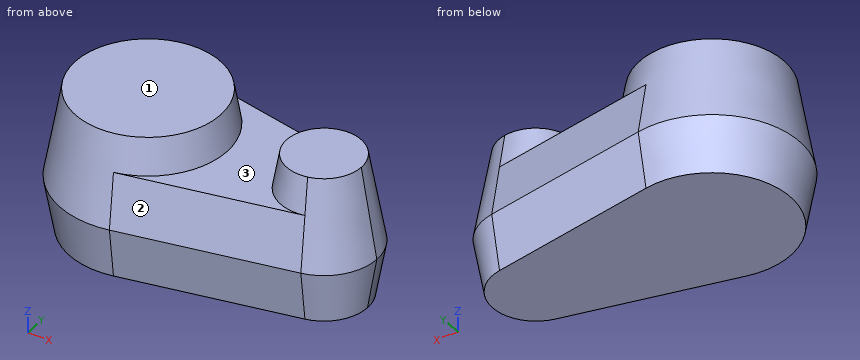
from build123d import *

# Parameters (mm, degrees)
F1_DEPTH = 50
F1_TAPER = 10
F2_DEPTH = 30
F2_TAPER = 10


with BuildPart() as f1:
    # F0 (on Top) → F1 (new body)
    with BuildSketch(Plane.XY):
        with BuildLine():
            ThreePointArc((10, -48.9897948557), (38.7298334621, -31.6227766017), (50, 0))
            ThreePointArc((50, 0), (38.7298334621, 31.6227766017), (10, 48.9897948557))
            ThreePointArc((10, 48.9897948557), (-50, 0), (10, -48.9897948557))
        make_face()
    extrude(amount=F1_DEPTH, taper=F1_TAPER)



with BuildPart() as f1b:
    # F0 (on Top) → F1, piece 2 (new body)
    with BuildSketch(Plane.XY):
        with BuildLine():
            ThreePointArc((130, 0), (123.2379000772, 18.973665961), (106, 29.3938769134))
            ThreePointArc((106, 29.3938769134), (70, 0), (106, -29.3938769134))
            ThreePointArc((106, -29.3938769134), (123.2379000772, -18.973665961), (130, 0))
        make_face()
    extrude(amount=F1_DEPTH, taper=F1_TAPER)


with BuildPart() as f1_1:
    add(f1.part)

    add(f1b.part)  # F2 merges F1b
    # F0 (on Top) → F2 (join, symmetric)
    with BuildSketch(Plane.XY):
        with BuildLine():
            ThreePointArc((10, 48.9897948557), (38.7298334621, 31.6227766017), (50, 0))
            ThreePointArc((50, 0), (38.7298334621, -31.6227766017), (10, -48.9897948557))
            Line((10, -48.9897948557), (106, -29.3938769134))
            ThreePointArc((106, -29.3938769134), (70, 0), (106, 29.3938769134))
            Line((106, 29.3938769134), (10, 48.9897948557))
        make_face()
        with BuildLine():
            ThreePointArc((10, -48.9897948557), (38.7298334621, -31.6227766017), (50, 0))
            ThreePointArc((50, 0), (38.7298334621, 31.6227766017), (10, 48.9897948557))
            ThreePointArc((10, 48.9897948557), (-50, 0), (10, -48.9897948557))
        make_face()
        with BuildLine():
            ThreePointArc((130, 0), (123.2379000772, 18.973665961), (106, 29.3938769134))
            ThreePointArc((106, 29.3938769134), (70, 0), (106, -29.3938769134))
            ThreePointArc((106, -29.3938769134), (123.2379000772, -18.973665961), (130, 0))
        make_face()
    extrude(amount=F2_DEPTH, both=True, taper=F2_TAPER)


solid = f1_1.part
Could you check a few things on this model? Use its own coordinates, in mm. Face numbers are marked on the shaded views. Round coordinates to 2 decimals unless told otherwise and drop trailing zeros. Write each loop counter-clockwise with the first axis right and the second up, starting at its lowest first coordinate (ties: lowest second). Pieces come first, ordered by that corner, then holes. Notation, with made-up numbers: (23.5, 10.25) -> (70.5, 10.25) arc R16 ccw to (70.5, 19.25) -> close; hole circle Ø5 at (44.5, 48). An arc over 180 degrees is marked (long way). Use a Markdown table: item, result.
1. If we section it at C-C (z = 12): List the corners of the cut face in (x, y) for me.
Answer key:
| item | result |
|---|---|
| outline | (9.58, -46.92) -> (105.58, -27.32) arc R27.88 ccw to (105.58, 27.32) -> (9.58, 46.92) arc R47.88 ccw (long way) to start |
2. We'd pull the mould along X, two halves only. Please class the marked faces 1, 2 and 3: +X half, -X half, draft (parallel to the pull), parting line (faces both ways), or undercut.
Answer key:
| item | result |
|---|---|
| face 1 | draft |
| face 2 | +X half |
| face 3 | undercut |
3. If we section it at A-A (x = 0): List the corners of the cut face in (y, z) for me.
Answer key:
| item | result |
|---|---|
| outline | (-50, 0) -> (-44.71, -30) -> (44.71, -30) -> (50, 0) -> (41.18, 50) -> (-41.18, 50) -> close |
4. If we section it at B-B (z = 37): List the corners of the cut face in (x, y) for me, then the cut area to 3 significant figures.
Answer key:
| item | result |
|---|---|
| outline | circle Ø86.95 at (0, 0); circle Ø46.95 at (100, 0) |
| area | 7,670 mm^2 |
5. Please list where these lines run through material, in increasing order: probe 1 along Z at (x, y) = (87.5, 25); probe 2 along X at (y, z) = (-8.5, 46); probe 3 along X at (y, z) = (-6, 37.5) (3 decimals).
Answer key:
| item | result |
|---|---|
| probe 1 | z = -30 to 30 |
| probe 2 | x = -41.02 to 41.02, 79.83 to 120.17 |
| probe 3 | x = -42.971 to 42.971, 77.395 to 122.605 |
6. For pin 1 Ø4 at (x, y) = (92, 26.5) entering from +Z; pin 2 Ø12 at (y, z) = (-20.5, 39.5) entering from -X; pin 3 Ø10 at (x, z) = (32.5, 14) entering from -Y, each with a flat end and sliding along its axis, tell me the tip position at first contact or that it passes through.
Answer key:
| item | result |
|---|---|
| pin 1 | stops at z = 30 |
| pin 2 | stops at x = -40.79 |
| pin 3 | stops at y = -43.24 |
